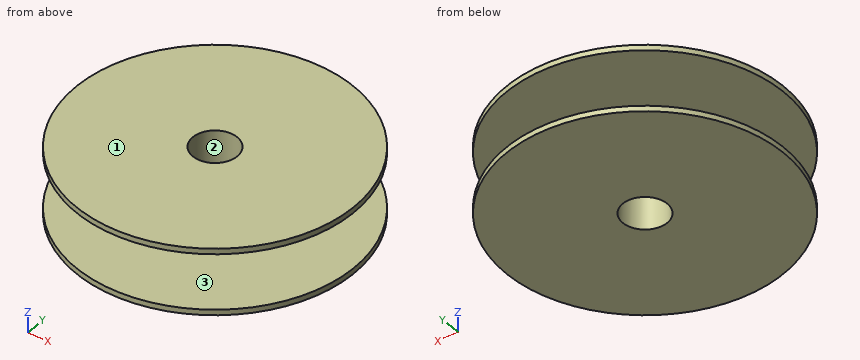
from build123d import *

# Parameters (mm, degrees)
SKETCH1_R           = 125
SKETCH1_R_2         = 20
BOSS_EXTRUDE1_DEPTH = 60
SHELL1_T            = -5


with BuildPart() as part:
    # Sketch1 → Boss-Extrude1 (new body)
    with BuildSketch(Plane.XY):
        Circle(SKETCH1_R)
        Circle(SKETCH1_R_2, mode=Mode.SUBTRACT)
    extrude(amount=BOSS_EXTRUDE1_DEPTH)

    # Shell1
    shell1_openings = [part.faces().sort_by_distance(p)[0] for p in [
        (-125, 0, 30),
    ]]
    offset(amount=SHELL1_T, openings=shell1_openings, kind=Kind.INTERSECTION)


solid = part.part
Source: CAD feature listing. Evaluate the final solid. Frame: model axes, mm. Face numbers are marked on the shaded views. Coordinates: 2 decimals unless noted, no trailing zeros. Loops run counter-clockwise (first coordinate to the right, second up) from the corner with the lowest first, then second, coordinate; pieces in that order, holes last. Notation, with made-up numbers: (64.25, -8) - (112.25, -8) arc R10 cw to (112.25, -2) - close; hole circle Ø9 at (-6.75, -39). An arc over 180 degrees is marked (long way). One line per item, written item: value. Start each with the question number.
1. Ray query, L1, parallel to Y at x = 0, z = 29; L2, parallel to Z at x = 40.5, y = 26. Return the intervals inside material, ascending.
2. Mould query, pull axis Z, two halves, no side actions, for the marked faces 1, 2 and 3. Classes: pulls with the +Z half, pulls with the -Z half, needs draft (parallel to the pull), parting line crosses it, or undercut.
3. Section A-A (x = 74.5). Return the cut outline in (y, z), and give its area (3 significant figures).
4. Section B-B (y = 0). Return the cut outline in (x, z).
5. Section D-D (z = 8). Return the cut outline in (x, y).
6. Section C-C (x = -6.5). Return the cut outline in (y, z), and give its area (3 significant figures).
7. Contact query for flat-ended pins moving along their axis: P1, Ø4, axis at x = -11, z = 22.5, coming from the -Y side; P2, Ø12, axis at y = -63, z = 48.5, coming from the +X side; P3, Ø2, axis at x = -20.5, z = 47, coming from the +Y side. Output: stop coordinate, or through.
Verdict:
1. L1: y = -25 to -20, 20 to 25
1. L2: z = 0 to 5, 55 to 60
2. face 1: pulls with the +Z half
2. face 2: needs draft
2. face 3: undercut
3. outline: (-100.37, 0) - (100.37, 0) - (100.37, 5) - (-100.37, 5) - close; (-100.37, 55) - (100.37, 55) - (100.37, 60) - (-100.37, 60) - close
3. area: 2,010 mm2
4. outline: (-125, 0) - (-20, 0) - (-20, 60) - (-125, 60) - (-125, 55) - (-25, 55) - (-25, 5) - (-125, 5) - close; (20, 0) - (125, 0) - (125, 5) - (25, 5) - (25, 55) - (125, 55) - (125, 60) - (20, 60) - close
5. outline: circle Ø50 at (0, 0); hole circle Ø40 at (0, 0)
6. outline: (-124.83, 0) - (-18.91, 0) - (-18.91, 60) - (-124.83, 60) - (-124.83, 55) - (-24.14, 55) - (-24.14, 5) - (-124.83, 5) - close; (18.91, 0) - (124.83, 0) - (124.83, 5) - (24.14, 5) - (24.14, 55) - (124.83, 55) - (124.83, 60) - (18.91, 60) - close
6. area: 2,640 mm2
7. P1: stops at y = -23.32
7. P2: passes through
7. P3: stops at y = 15.64
